Part model, mm, in its own coordinate system. A direction names the side the tool comes from. Coordinates: 2 decimals unless noted, no trailing zeros. Write each loop counter-clockwise with the first axis right and the second up, starting at its lowest first coordinate (ties: lowest second). Pieces come first, ordered by that corner, then holes. Notation, with made-up numbers: (7, -35.5) -> (26, -35.5) arc R13 ccw to (26, -19.5) -> close; hole circle Ø8 at (88, -39.75). An arc over 180 degrees is marked (long way). One line per question, with ' | ' between items. Start each with the question number.
Item 1: Saw through at C-C (x = 9). List the corners of the cut face in (y, z).
Item 2: Saw through at B-B (y = 0.5). List the corners of the cut face in (x, z), and give its area (3 significant figures).
Item 3: Probe probe 1 along Y at (x, z) = (17, 5.5); probe 2 along X at (y, z) = (24, 34); probe 3 along Y at (x, z) = (16.65, 1.4). List the from-to ranges inside material, lowest first. Write a range as [from, to].
Item 4: Two-plate mould, pull along Y, no slides. Class faces 1 (the flat face through (27.5, 0, 21)), 2 (the cylindrical face through (-22.1, 22.07, 23.27)), 3 (the flat face through (0, -27.5, 21)): pulls with the +Y half, pulls with the -Y half, needs draft (parallel to the pull), parting line crosses it, or undercut.
Item 5: 3-axis set-ups, long thin cutter, end or side, ignore diameter. For faces 4 (the flat face through (-25, 25, 32)), 5 (the cylindrical face through (-26.64, -26.6, 21.79)): which of +Z, -Z, +X, -X, +Y, -Y reach the whole face in a straight line?
Item 6: Pin check, flat tips, straight feed: pin 1 (1.8 mm diameter, centred on x = 16.65, y = 16.65, fed in from -Z); pin 2 (0.8 mm diameter, centred on x = 24, y = -24.5, fed in from +Z). Stop position of each tip, or through.
Item 7: Saw through at D-D (y = 16.65). List the corners of the cut face in (x, z).
from build123d import *

# Parameters (mm, degrees)
F0_W     = 55
F0_H     = 55
F0_R     = 1.5
F0_R_2   = 18.75
F1_DEPTH = 2
F2_W     = 55
F2_H     = 55
F3_DEPTH = 40
F4_R     = 1.25
F5_DEPTH = 10
F6_R     = 3
F7_R     = 1
F8_F1_R  = 2
F8_F2_R  = 1.9999


# Not quite as in the source:
# - a fillet or chamfer is up to 0.001 mm smaller than in the source, because OpenCascade refuses the exact size


with BuildPart() as f1:
    # F0 (on Top) → F1 (new body)
    with BuildSketch(Plane.XY):
        Rectangle(F0_W, F0_H)
        with Locations((-16.65, -16.65)):
            Circle(F0_R, mode=Mode.SUBTRACT)
        with Locations((16.65, -16.65)):
            Circle(F0_R, mode=Mode.SUBTRACT)
        with Locations((-16.65, 16.65)):
            Circle(F0_R, mode=Mode.SUBTRACT)
        with Locations((0, 0.5)):
            Circle(F0_R_2, mode=Mode.SUBTRACT)
        with Locations((16.65, 16.65)):
            Circle(F0_R, mode=Mode.SUBTRACT)
    extrude(amount=F1_DEPTH)

    # F2 (on face) → F3 (join)
    with BuildSketch(Plane.XY.offset(2)):
        Rectangle(F2_W, F2_H)
        Polygon((-21.5, 21.5), (-21.5, 25.5), (21.5, 25.5), (21.5, 21.5), (25.5, 21.5), (25.5, -21.5), (21.5, -21.5), (21.5, -25.5), (-21.5, -25.5), (-21.5, -21.5), (-25.5, -21.5), (-25.5, 21.5), align=None, mode=Mode.SUBTRACT)
    extrude(amount=F3_DEPTH)

    # F4 (on face) → F5 (cut)
    with BuildSketch(Plane.XY.offset(42)):
        with Locations((-24.5, 24.5)):
            Circle(F4_R)
        with Locations((-24.5, -24.5)):
            Circle(F4_R)
        with Locations((24.5, -24.5)):
            Circle(F4_R)
        with Locations((24.5, 24.5)):
            Circle(F4_R)
    extrude(amount=-F5_DEPTH, mode=Mode.SUBTRACT)

    # F6
    f6_edges = [f1.edges().sort_by_distance(p)[0] for p in [
        (-27.5, -27.5, 21),
        (27.5, -27.5, 21),
        (-27.5, 27.5, 21),
        (27.5, 27.5, 21),
    ]]
    fillet(f6_edges, radius=F6_R)

    # F7
    f7_edges = [f1.edges().sort_by_distance(p)[0] for p in [
        (0, -27.5, 0),
        (27.5, 0, 0),
        (26.62132, -26.62132, 0),
        (26.62132, 26.62132, 0),
        (0, 27.5, 0),
        (-26.62132, -26.62132, 0),
        (-26.62132, 26.62132, 0),
        (-27.5, 0, 0),
    ]]
    fillet(f7_edges, radius=F7_R)

    # F8: fillet of radius 2 on 20 edges, made by hand

    # F8_f1
    f8_f1_edges = [f1.edges().sort_by_distance(p)[0] for p in [
        (21.5, -21.5, 22),
        (-21.5, -21.5, 22),
        (-21.5, 21.5, 22),
        (21.5, 21.5, 22),
    ]]
    fillet(f8_f1_edges, radius=F8_F1_R)

    # F8_f2 (radius 2 in the source; OpenCascade refuses exactly that, so slightly less here)
    f8_f2_edges = [f1.edges().sort_by_distance(p)[0] for p in [
        (-21.5, -25.5, 22),
        (-25.5, -21.5, 22),
        (21.5, -25.5, 22),
        (25.5, -21.5, 22),
        (-25.5, 21.5, 22),
        (-21.5, 25.5, 22),
        (21.5, 25.5, 22),
        (25.5, 21.5, 22),
        (0, -25.5, 2),
        (25.5, 0, 2),
        (-25.5, 0, 2),
        (0, 25.5, 2),
        (-24.5, -21.5, 2),
        (-21.5, 24.5, 2),
        (21.5, -24.5, 2),
        (24.5, 21.5, 2),
        (22.0857864376, 22.0857864376, 2),
        (22.0857864376, -22.0857864376, 2),
        (-22.0857864376, 22.0857864376, 2),
        (-22.0857864376, -22.0857864376, 2),
    ]]
    fillet(f8_f2_edges, radius=F8_F2_R)


solid = f1.part
From the geometry:
1) outline: (-27.5, 1) arc R1 ccw to (-26.5, 0) -> (-15.95, 0) -> (-15.95, 2) -> (-23.5, 2) arc R2 cw to (-25.5, 4) -> (-25.5, 42) -> (-27.5, 42) -> close; (16.95, 0) -> (26.5, 0) arc R1 ccw to (27.5, 1) -> (27.5, 42) -> (25.5, 42) -> (25.5, 4) arc R2 cw to (23.5, 2) -> (16.95, 2) -> close
2) outline: (-27.5, 1) arc R1 ccw to (-26.5, 0) -> (-18.75, 0) -> (-18.75, 2) -> (-23.5, 2) arc R2 cw to (-25.5, 4) -> (-25.5, 42) -> (-27.5, 42) -> close; (18.75, 0) -> (26.5, 0) arc R1 ccw to (27.5, 1) -> (27.5, 42) -> (25.5, 42) -> (25.5, 4) arc R2 cw to (23.5, 2) -> (18.75, 2) -> close | area: 196 mm2
3) probe 1: [-27.5, -25.5], [25.5, 27.5] | probe 2: [-27.5, -25.65], [-23.35, -21.44], [21.44, 23.35], [25.65, 27.5] | probe 3: [-27.5, -18.15], [-15.15, -8.12], [9.12, 15.15], [18.15, 27.5]
4) face 1: needs draft | face 2: undercut | face 3: pulls with the -Y half
5) face 4: +Z | face 5: +Z, -Z, -X, -Y
6) pin 1: through | pin 2: z = 32
7) outline: (-27.5, 1) arc R1 ccw to (-26.5, 0) -> (-18.15, 0) -> (-18.15, 2) -> (-23.5, 2) arc R2 cw to (-25.5, 4) -> (-25.5, 42) -> (-27.5, 42) -> close; (-15.15, 0) -> (-9.53, 0) -> (-9.53, 2) -> (-15.15, 2) -> close; (9.53, 0) -> (15.15, 0) -> (15.15, 2) -> (9.53, 2) -> close; (18.15, 0) -> (26.5, 0) arc R1 ccw to (27.5, 1) -> (27.5, 42) -> (25.5, 42) -> (25.5, 4) arc R2 cw to (23.5, 2) -> (18.15, 2) -> close
